from build123d import *

# Parameters (mm, degrees)
F0_R        = 37.981107
F0_R_2      = 21.625719
F1_DEPTH    = 42.926
F1_FACE_R   = 37.981107
F1_FACE_R_2 = 21.625719
F2_DEPTH    = 14.224
F3_DEPTH    = 25.4


with BuildPart() as f1:
    # F0 (on Top) → F1 (new body)
    with BuildSketch(Plane.XY):
        Circle(F0_R)
        with Locations((-10.219174, 0)):
            Circle(F0_R_2, mode=Mode.SUBTRACT)
    extrude(amount=F1_DEPTH)

    # F1_face (on face) → F2 (cut)
    with BuildSketch(Plane(origin=(4.902302, 0, 42.926), x_dir=(1, 0, 0), z_dir=(0, 0, 1))):
        with Locations((-4.902302, 0)):
            Circle(F1_FACE_R)
        with Locations((-15.121476, 0)):
            Circle(F1_FACE_R_2, mode=Mode.SUBTRACT)
    extrude(amount=F2_DEPTH, mode=Mode.SUBTRACT)

    # F1_face (on face) → F3 (join)
    with BuildSketch(Plane(origin=(4.902302, 0, 42.926), x_dir=(1, 0, 0), z_dir=(0, 0, 1))):
        with Locations((-4.902302, 0)):
            Circle(F1_FACE_R)
        with Locations((-15.121476, 0)):
            Circle(F1_FACE_R_2, mode=Mode.SUBTRACT)
    extrude(amount=F3_DEPTH)


solid = f1.part
Geometry check sheet. Reference: the model listing, model coordinates, mm. Round coordinates to 2 decimals unless told otherwise and drop trailing zeros. Loops run counter-clockwise (first coordinate to the right, second up) from the corner with the lowest first, then second, coordinate; pieces in that order, holes last.
Item 1: Cross-section at D-D on x = 28. Record the boundary of the cut face in (y, z).
Item 2: Thickness scan on line 1 (X direction, y = -15.5, z = 17.5); line 2 (Y direction, x = -29.5, z = 61.5); line 3 (Y direction, x = 4, z = 56). Record the ranges inside material, lowest first.
Item 3: Cross-section at B-B on x = -27.5. Record the boundary of the cut face in (y, z).
Item 4: Cross-section at C-C on z = 33. Record the boundary of the cut face in (x, y), then the cut area to 3 significant figures.
Item 5: Cross-section at A-A on y = 0. Record the boundary of the cut face in (x, z), then the cut area to 4 significant figures.
Item 6: Mould release check, pull along X, two halves, no side actions. Record for faces 1 (the cylindrical face through (-14.91, -21.11, 33.68)), 2 (the flat face through (16, 1, 0)), 3 (the cylindrical face through (36.227, 11.408, 33.685)): pulls with the +X half, pulls with the -X half, needs draft (parallel to the pull), parting line crosses it, or undercut.
Item 7: Gauge pin test, flat ends, axial feed: pin 1 (5 mm diameter, centred on x = -8.5, z = 23, fed in from -Y); pin 2 (5 mm diameter, centred on y = -12.5, z = 44, fed in from +X); pin 3 (6 mm diameter, centred on x = -1.5, z = 51, fed in from -Y). Record the tip position at first contact, or that the pin passes through.
Answer sheet:
1. outline: (-25.66, 0) - (25.66, 0) - (25.66, 68.33) - (-25.66, 68.33) - close
2. line 1: x = -34.67 to -25.3, 4.86 to 34.67
2. line 2: y = -23.92 to -9.79, 9.79 to 23.92
2. line 3: y = -37.77 to -16.29, 16.29 to 37.77
3. outline: (-26.2, 0) - (-13, 0) - (-13, 68.33) - (-26.2, 68.33) - close; (13, 0) - (26.2, 0) - (26.2, 68.33) - (13, 68.33) - close
4. outline: circle Ø75.96 at (0, 0); hole circle Ø43.25 at (-10.22, 0)
4. area: 3,060 mm2
5. outline: (-37.98, 0) - (-31.84, 0) - (-31.84, 68.33) - (-37.98, 68.33) - close; (11.41, 0) - (37.98, 0) - (37.98, 68.33) - (11.41, 68.33) - close
5. area: 2,235 mm2
6. face 1: undercut
6. face 2: needs draft
6. face 3: parting line crosses it
7. pin 1: stops at y = -37.5
7. pin 2: stops at x = 36.64
7. pin 3: stops at y = -37.98
